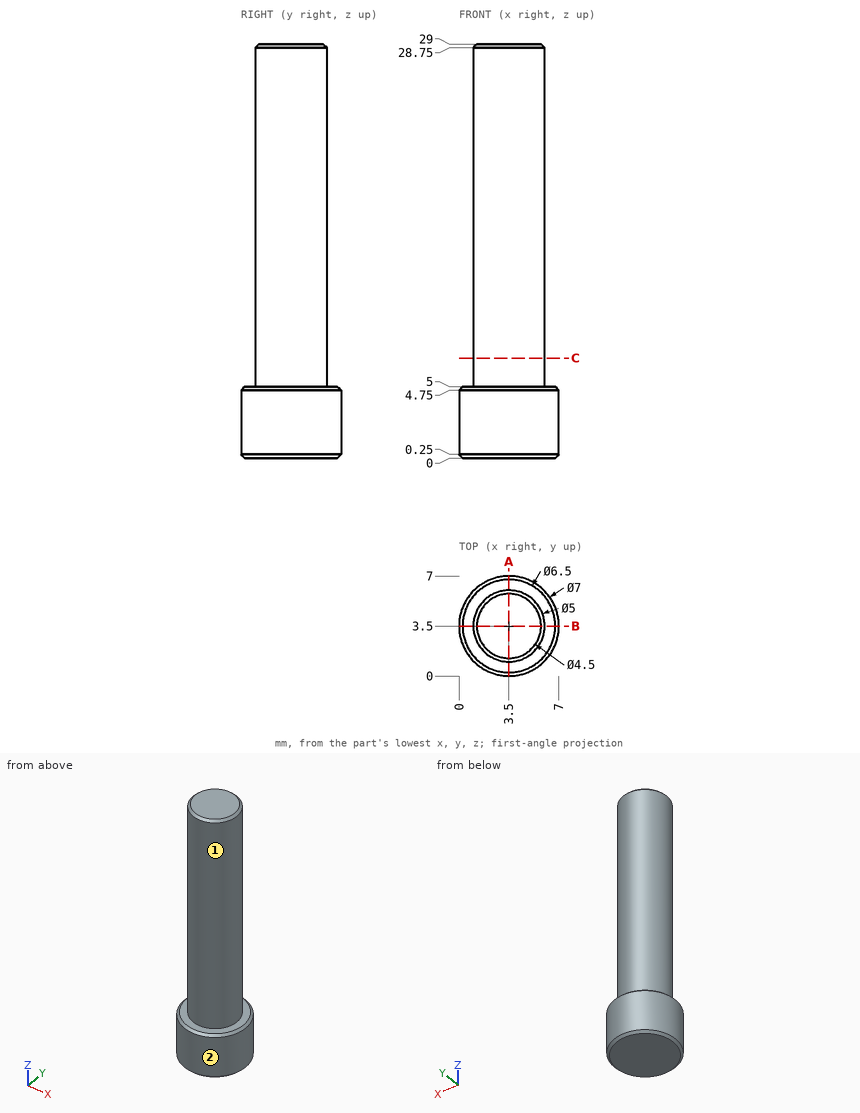
Source: three-view drawing plus pictorial views. Frame: mm from the lowest corner of the part. A direction names the side the tool comes from. Round coordinates to 2 decimals unless told otherwise and drop trailing zeros. Loops run counter-clockwise (first coordinate to the right, second up) from the corner with the lowest first, then second, coordinate; pieces in that order, holes last. Notation, with made-up numbers: M 26,49 L 84,49 A24 ccw 84,70 Z; hole C 39,1 d3. An arc over 180 degrees is marked long. Put each result on its own line as item: value. Start each with the question number.
(1) Material intervals for line 1 along Z through (x, y) = (3.5, 6.5); line 2 along Y through (x, z) = (3.5, 20); line 3 along Z through (x, y) = (5.25, 2), sorted ascending. Write a range as [from, to].
(2) Section query A-A (x = 3.5). Return loops of the section in (y, z), then the cut area to 3 significant figures.
(3) Set-up query: the marked faces 1 and 2. Return all of +Z, -Z, +X, -X, +Y, -Y with unobstructed straight access to the full face (end or side cutting, diameter ignored); none if empty.
(4) Section query C-C (z = 7). Return loops of the section in (x, y).
(5) Contact query for flat-ended pins moving along their axis: pin 1 Ø1.5 at (x, y) = (6, 2.5) entering from -Z; pin 2 Ø4 at (x, z) = (1, 11.5) entering from +Y. Output: stop coordinate, or through.
Findings below:
1. line 1: z = [0, 5]
1. line 2: y = [1, 6]
1. line 3: z = [0, 28.95]
2. outline: M 0,0.25 L 0.25,0 L 6.75,0 L 7,0.25 L 7,4.75 L 6.75,5 L 6,5 L 6,28.75 L 5.75,29 L 1.25,29 L 1,28.75 L 1,5 L 0.25,5 L 0,4.75 Z
2. area: 155 mm2
3. face 1: +Z
3. face 2: +Z, -Z
4. outline: C 3.5,3.5 d5
5. pin 1: stops at z = 0
5. pin 2: stops at y = 5.95
